Source: CAD feature listing. Evaluate the final solid. Frame: model axes, mm. A direction names the side the tool comes from. Give positions to 0.01 mm unless a question says otherwise; leave off trailing zeros. Order: outer loops, then holes, each group sorted by start corner. A loop starts at its lowest first (then second) coordinate and runs counter-clockwise, first axis right, second up. Notation, with made-up numbers: (-25.75, 4) -> (-8.75, 4) arc R14 cw to (-8.75, 22) -> close; hole circle Ø11 at (8, 47.5). An arc over 180 degrees is marked (long way). Use CSV: the item, a comma, the result in double quotes.
```python
from build123d import *

# Parameters (mm, degrees)
SKETCH1_R           = 12.5
BOSS_EXTRUDE1_DEPTH = 19
SKETCH2_R           = 12.1
BOSS_EXTRUDE2_DEPTH = 31
BOSS_EXTRUDE3_DEPTH = 14
SKETCH4_W           = 3.8
SKETCH4_H           = 10.4
BOSS_EXTRUDE4_DEPTH = 5
SKETCH5_R           = 3.5
BOSS_EXTRUDE5_DEPTH = 2.7
SKETCH6_R           = 2
BOSS_EXTRUDE6_DEPTH = 12.3
SKETCH7_R           = 1.5
CUT_EXTRUDE1_DEPTH  = 5


with BuildPart() as part:
    # Sketch1 → Boss-Extrude1 (new body)
    with BuildSketch(Plane.XY):
        Circle(SKETCH1_R)
    extrude(amount=BOSS_EXTRUDE1_DEPTH)

    # Sketch2 → Boss-Extrude2 (add)
    with BuildSketch(Plane.XY.offset(19)):
        Circle(SKETCH2_R)
    extrude(amount=BOSS_EXTRUDE2_DEPTH)

    # Sketch3 → Boss-Extrude3 (add)
    with BuildSketch(Plane.XY.offset(50)):
        with BuildLine():
            Line((-12.1, 0), (-12.1, 19.9))
            Line((-12.1, 19.9), (12.1, 19.9))
            Line((12.1, 19.9), (12.1, 0))
            ThreePointArc((12.1, 0), (0, -12.1), (-12.1, 0))
        make_face()
    extrude(amount=BOSS_EXTRUDE3_DEPTH)

    # Sketch4 → Boss-Extrude4 (add)
    with BuildSketch(Plane(origin=(0, 0, 50), x_dir=(-1, 0, 0), z_dir=(0, 0, -1))):
        with Locations((-10.1, 14.6)):
            Rectangle(SKETCH4_W, SKETCH4_H)
    extrude(amount=BOSS_EXTRUDE4_DEPTH)

    # Sketch5 → Boss-Extrude5 (add)
    with BuildSketch(Plane(origin=(0, 0, 0), x_dir=(-1, 0, 0), z_dir=(0, 0, -1))):
        with Locations(Location((0, 0, 0), (0, 0, 180))):
            Circle(SKETCH5_R)
    extrude(amount=BOSS_EXTRUDE5_DEPTH)

    # Sketch6 → Boss-Extrude6 (add)
    with BuildSketch(Plane(origin=(0, 0, 0), x_dir=(-1, 0, 0), z_dir=(0, 0, -1))):
        Circle(SKETCH6_R)
    extrude(amount=BOSS_EXTRUDE6_DEPTH)

    # Sketch7 → Cut-Extrude1 (cut)
    with BuildSketch(Plane(origin=(0, 0, 0), x_dir=(-1, 0, 0), z_dir=(0, 0, -1))):
        with Locations((6.01040764, 6.01040764)):
            Circle(SKETCH7_R)
        with Locations((-6.01040764, -6.01040764)):
            Circle(SKETCH7_R)
    extrude(amount=-CUT_EXTRUDE1_DEPTH, mode=Mode.SUBTRACT)


solid = part.part
```
1. Section query A-A on x = 0. Return loops of the section in (y, z).
Answer below:
outline,"(-12.5, 0) -> (-3.5, 0) -> (-3.5, -2.7) -> (-2, -2.7) -> (-2, -12.3) -> (2, -12.3) -> (2, -2.7) -> (3.5, -2.7) -> (3.5, 0) -> (12.5, 0) -> (12.5, 19) -> (12.1, 19) -> (12.1, 50) -> (19.9, 50) -> (19.9, 64) -> (-12.1, 64) -> (-12.1, 19) -> (-12.5, 19) -> close"
2. Section query B-B on y = -10. Return loops of the section in (x, z).
Answer below:
outline,"(-7.5, 0) -> (7.5, 0) -> (7.5, 19) -> (6.81, 19) -> (6.81, 64) -> (-6.81, 64) -> (-6.81, 19) -> (-7.5, 19) -> close"
3. Section query C-C on z = 36. Return loops of the section in (x, y), plus the area to 3 significant figures.
Answer below:
outline,"circle Ø24.2 at (0, 0)"
area,"460 mm²"
4. Access query for faces 4 (the cylindrical face through (-1.575, -11.997, 36.185)), 5 (the flat face through (10, 19.8, 48)), 6 (the flat face through (10, 15, 45)), 7 (the flat face through (6, -6, 5)), 8 (the flat face through (0, 4, 64)). Directions: +Z, -Z, +X, -X, +Y, -Y. A direction counts if a zero-diameter tool reaches every point of the face in a straight line with its end or side. Return the directions, or none.
Answer below:
face 4,"none"
face 5,"-Z, +X, -X, +Y"
face 6,"-Z, +X, +Y"
face 7,"-Z"
face 8,"+Z, +X, -X, +Y, -Y"
5. Section query D-D on z = 2.5. Return loops of the section in (x, y), plus the area to 3 significant figures.
Answer below:
outline,"circle Ø25 at (0, 0); hole circle Ø3 at (-6.01, 6.01); hole circle Ø3 at (6.01, -6.01)"
area,"477 mm²"
6. Pin query (flat end, axial travel): P1, Ø3.5, axis at x = 5.5, y = -5.5, coming from the -Z side; P2, Ø4, axis at y = 13.5, z = 46.5, coming from the +X side; P3, Ø1.1, axis at x = 9.5, z = 47.5, coming from the -Y side. Return the tip coordinate at first contact, or that it passes through.
Answer below:
P1,"stops at z = 0"
P2,"stops at x = 12"
P3,"stops at y = -8.14"
7. Ray query, line 1 along X through (y, z) = (14, 52.5); line 2 along Z through (x, y) = (-5, 16); line 3 along Z through (x, y) = (1, 5). Return the intervals inside material, ascending.
Answer below:
line 1,"x = -12.1 to 12.1"
line 2,"z = 50 to 64"
line 3,"z = 0 to 64"
8. Mould query, pull axis Y, two halves, no side actions, for faces 1 (the cylindrical face through (3.233, 1.341, -1.331)), 2 (the cylindrical face through (-7.396, 5.436, 2.465)), 3 (the flat face through (12.1, 10, 57)). Classes: released by +Y, released by -Y, zero draft, split by the parting line, or undercut.
Answer below:
face 1,"split by the parting line"
face 2,"undercut"
face 3,"zero draft"
